from build123d import *

# Parameters (mm, degrees)
BOSS_EXTRUDE1_DEPTH = 13
SKETCH1_3_R         = 5
SKETCH1_3_R_2       = 2
BOSS_EXTRUDE2_DEPTH = 1
SKETCH1_5_W         = 2
SKETCH1_5_H         = 9.797958972
BOSS_EXTRUDE3_DEPTH = 20


with BuildPart() as part:
    # Sketch1 → Boss-Extrude1 (new body)
    with BuildSketch(Plane(origin=(0, 0, 0), x_dir=(1, 0, 0), z_dir=(0, 1, 0))):
        with BuildLine():
            Line((2.5, 2.5), (2.5, -2.5))
            ThreePointArc((2.5, -2.5), (0, -5), (-2.5, -2.5))
            Line((-2.5, -2.5), (-2.5, 2.5))
            ThreePointArc((-2.5, 2.5), (0, 5), (2.5, 2.5))
        make_face()
    extrude(amount=-BOSS_EXTRUDE1_DEPTH)

    # Sketch1_3 → Boss-Extrude2 (add)
    with BuildSketch(Plane(origin=(0, 0, 0), x_dir=(1, 0, 0), z_dir=(0, 1, 0))):
        Circle(SKETCH1_3_R)
        with Locations((0.435778714, -4.98097349)):
            Circle(SKETCH1_3_R_2)
        with Locations((-4.98097349, 0.435778714)):
            Circle(SKETCH1_3_R_2)
        with Locations((3.535533906, 3.535533906)):
            Circle(SKETCH1_3_R_2)
    extrude(amount=-BOSS_EXTRUDE2_DEPTH)

    # Sketch1_5 → Boss-Extrude3 (add)
    with BuildSketch(Plane(origin=(0, 0, 0), x_dir=(1, 0, 0), z_dir=(0, 1, 0))):
        Rectangle(SKETCH1_5_W, SKETCH1_5_H)
    extrude(amount=BOSS_EXTRUDE3_DEPTH)


solid = part.part
Verification items for the finished model (mm, model axes). A direction names the side the tool comes from. Coordinates: 2 decimals unless noted, no trailing zeros. Write each loop counter-clockwise with the first axis right and the second up, starting at its lowest first coordinate (ties: lowest second). Pieces come first, ordered by that corner, then holes. Notation, with made-up numbers: M 82.5,25 L 117.5,25 A24 cw 117.5,49 Z; hole C 74.5,-24 d8. An arc over 180 degrees is marked long. Use a Markdown table: item, result.
Q1. Go/stop test with flat-tipped pins: P1, Ø6.5, axis at x = -3, z = 1, coming from the -Y side; P2, Ø2.5, axis at y = -5, z = 0.5, coming from the -X side; P3, Ø2, axis at x = 0, y = 8, coming from the -Z side; P4, Ø1.5, axis at y = -10, z = -0.5, coming from the +X side. Record where each tip stops, or that it passes through.
Reply:
| item | result |
|---|---|
| P1 | stops at y = -13 |
| P2 | stops at x = -2.5 |
| P3 | stops at z = -4.9 |
| P4 | stops at x = 2.5 |
Q2. Sectioned sample at C-C, the plane x = 4. Record the boundary of the cut face in (y, z).
Reply:
| item | result |
|---|---|
| outline | M -1,-5.48 L 0,-5.48 L 0,3 L -1,3 Z |
Q3. Sectioned sample at B-B, the plane y = 13.5. Record the boundary of the cut face in (x, z), plus the area to 3 significant figures.
Reply:
| item | result |
|---|---|
| outline | M -1,-4.9 L 1,-4.9 L 1,4.9 L -1,4.9 Z |
| area | 19.6 mm² |
Q4. Sectioned sample at A-A, the plane z = 4. Record the boundary of the cut face in (x, y), plus the area to 3 significant figures.
Reply:
| item | result |
|---|---|
| outline | M -3,-1 L -2,-1 L -2,-13 L 2,-13 L 2,-1 L 3,-1 L 3,0 L 1,0 L 1,20 L -1,20 L -1,0 L -3,0 Z |
| area | 94.0 mm² |
Q5. Thickness scan on line 1 (X direction, y = 11, z = 3.25); line 2 (Y direction, x = -4.75, z = 1); line 3 (X direction, y = -7.5, z = -0.5). Record the ranges inside material, lowest first.
Reply:
| item | result |
|---|---|
| line 1 | x = -1 to 1 |
| line 2 | y = -1 to 0 |
| line 3 | x = -2.5 to 2.5 |
Q6. Draft check along X on faces 1 (the face through (4.68, -0.49, 1.76)), 2 (the face through (2, 0, 1)), 3 (the face through (-1.662, -0.493, -4.716)). Enter one of: +X half, -X half, draft (parallel to the pull), parting line (faces both ways), or undercut.
Reply:
| item | result |
|---|---|
| face 1 | +X half |
| face 2 | draft |
| face 3 | undercut |
Q7. Set-up check for faces 4 (the face through (-2.5, -7, 0)), 5 (the face through (0, -7, 5)), 6 (the face through (-1, 10, 0)): record each of +Z, -Z, +X, -X, +Y, -Y from which the full face is reachable in a straight line by a thin tool's end or side.
Reply:
| item | result |
|---|---|
| face 4 | +Z, -Z, -X, -Y |
| face 5 | +Z, -Y |
| face 6 | +Z, -Z, -X, +Y |
Q8. Sectioned sample at D-D, the plane z = 1.25. Record the boundary of the cut face in (x, y), plus the area to 3 significant figures.
Reply:
| item | result |
|---|---|
| outline | M -6.06,-1 L -2.5,-1 L -2.5,-13 L 2.5,-13 L 2.5,-1 L 4.84,-1 L 4.84,0 L 1,0 L 1,20 L -1,20 L -1,0 L -6.06,0 Z |
| area | 111 mm² |
